Part model, mm, in its own coordinate system. A direction names the side the tool comes from. Give positions to 0.01 mm unless a question says otherwise; leave off trailing zeros. Answer in a Markdown table with one row per item. Add a question column.
1. Drop flat-ended pins along their axis: pin 1 Ø12 at (y, z) = (13, -27.5) entering from -X; pin 2 Ø2 at (x, y) = (-17, 9) entering from +Z; pin 3 Ø4 at (x, y) = (-11.5, 27.5) entering from +Z; pin 4 Ø1.5 at (x, z) = (-12.5, -30.5) entering from -Y. Give the stop position or say it passes through.
2. Probe line 1 along Z through (x, y) = (-9, 12); line 2 along X through (y, z) = (16, 34); line 3 along X through (y, z) = (32, 9). List the from-to ranges inside material, lowest first.
3. Band-saw the part on A-A on y = 12. State how many separate pieces and enclosed holes the cut face has, plus the area to 3 significant figures.
4. Which spindle directions (+Z, -Z, +X, -X, +Y, -Y) get a long thin tool onto all of the face, cutting with end or side? Do faces 1 (the flat face through (-3, 14, -25)), 2 (the flat face through (15, 15, -27)), 3 (the cylindrical face through (-24.08, 12.68, -13.28)), 4 (the flat face through (0, 25, 29)), 5 (the flat face through (0, 23, 30.35)). Say none if no direction does.
5. Pull direction Z, two halves, no side cores. Call faces 6 (the flat face through (3.61, 23.03, 32.45)), 7 (the flat face through (-15, 15, -27)), 8 (the conical face through (-1.036, 34.514, 24.386)): released by +Z, released by -Z, zero draft, split by the parting line, or undercut.
```python
from build123d import *

# Parameters (mm, degrees)
SKETCH2_W               = 6
SKETCH2_H               = 60
CUT_EXTRUDE1_DEPTH      = 67.520673478
CUT_EXTRUDE2_DEPTH      = 69.366658541
CUT_EXTRUDE2_DEPTH_BACK = 69.366658541
SKETCH3_R               = 4.25
SKETCH6_R               = 2.65
CUT_EXTRUDE5_DEPTH      = 67.520673599
CUT_EXTRUDE6_DEPTH      = 4
CUT_EXTRUDE7_DEPTH      = 62.846584554
FILLET1_R               = 28
SKETCH12_W              = 12
SKETCH12_H              = 3
BOSS_EXTRUDE1_DEPTH     = 25
CHAMFER1_SIZE           = 0.5
FILLET2_R               = 2
SKETCH13_R              = 4.625
CUT_EXTRUDE8_DEPTH      = 53.561734699
SKETCH15_R              = 2.65
BOSS_EXTRUDE2_DEPTH     = 0.2
SKETCH16_R              = 15
CUT_EXTRUDE9_DEPTH      = 55.660186193
FILLET3_R               = 11
FILLET4_R               = 24


with BuildPart() as part:
    # Sketch1 → Revolve1 (revolve)
    with BuildSketch(Plane.XY, mode=Mode.PRIVATE) as revolve1_sk:
        Polygon((16.25, 0), (40, 0), (40, 25), (27.5, 25), (24.25, 35), (16.25, 35), align=None)
    revolve(revolve1_sk.sketch.rotate(Axis((0, 0, 0), (0, 1, 0)), 90), axis=Axis((0, 0, 0), (0, 1, 0)))

    # Sketch2 → Cut-Extrude1 (cut, through all)
    with BuildSketch(Plane.XZ):
        with Locations((0, -30)):
            Rectangle(SKETCH2_W, SKETCH2_H)
    extrude(amount=-CUT_EXTRUDE1_DEPTH, mode=Mode.SUBTRACT)

    # Sketch3 → Cut-Extrude2 (cut, two sides: drawn at the far end of the back side and taken through both)
    with BuildSketch(Plane(origin=(-3, 0, 0), x_dir=(0, 0, -1), z_dir=(1, 0, 0)).offset(-CUT_EXTRUDE2_DEPTH_BACK)):
        with Locations((30.970676254, 12)):
            Circle(SKETCH3_R)
    extrude(amount=CUT_EXTRUDE2_DEPTH + CUT_EXTRUDE2_DEPTH_BACK, mode=Mode.SUBTRACT)

    # Sketch6 → Cut-Extrude5 (cut, through all)
    with BuildSketch(Plane.XZ):
        with Locations(Location((0, 34.5, 0), (0, 0, 270))):
            Circle(SKETCH6_R)
    extrude(amount=-CUT_EXTRUDE5_DEPTH, mode=Mode.SUBTRACT)

    # Sketch7 → Cut-Extrude6 (cut)
    with BuildSketch(Plane(origin=(0, 25, 0), x_dir=(1, 0, 0), z_dir=(0, 1, 0))):
        Polygon((-2.396003617, -30.35), (-4.792007234, -34.5), (-2.396003617, -38.65), (2.396003617, -38.65), (4.792007234, -34.5), (2.396003617, -30.35), align=None)
    extrude(amount=-CUT_EXTRUDE6_DEPTH, mode=Mode.SUBTRACT)

    # Sketch8 → Cut-Extrude7 (cut, through all)
    with BuildSketch(Plane(origin=(0, 25, 0), x_dir=(1, 0, 0), z_dir=(0, 1, 0))):
        with BuildLine():
            Line((-27.5, 0), (-27.5, -50))
            Line((-27.5, -50), (-50, -50))
            Line((-50, -50), (-50, 70))
            Line((-50, 70), (50, 70))
            Line((50, 70), (50, -50))
            Line((50, -50), (27.5, -50))
            Line((27.5, -50), (27.5, 0))
            ThreePointArc((27.5, 0), (24.173849507, 13.110110602), (15, 23.048861143))
            Line((15, 23.048861143), (15, 60))
            Line((15, 60), (-15, 60))
            Line((-15, 60), (-15, 23.048861143))
            ThreePointArc((-15, 23.048861143), (-24.173849507, 13.110110602), (-27.5, 0))
        make_face()
    extrude(amount=-CUT_EXTRUDE7_DEPTH, mode=Mode.SUBTRACT)

    # Fillet1
    # the kernel refuses this fillet: 28 mm, written as the material it takes off along each edge
    with BuildSketch(Plane(origin=(27.5, -77.857831737, 29.047375097), x_dir=(-0.9365360560407987, 0, 0.3505712705507198), z_dir=(0, 1, 0))) as fillet1_piece_1:
        with BuildLine():
            CenterArc((20.243036252, -25.791236836), FILLET1_R, 67.089723989, 92.388015463)
            Line((-5.979973318, -15.975241261), (0, 0))
            ThreePointArc((0, 0), (15.571566347, 3.155375949), (31.143132695, 0))
        make_face()
    extrude(amount=180.715663474, mode=Mode.SUBTRACT)
    with BuildSketch(Plane(origin=(-27.5, -77.857831737, 29.047375097), x_dir=(0, 0, -1), z_dir=(0, 1, 0))) as fillet1_piece_2:
        with BuildLine():
            CenterArc((17.057796288, -28), FILLET1_R, 90, 92.388015463)
            ThreePointArc((-10.917887598, -29.166666667), (-8.414067145, -13.477149178), (0, 0))
            Line((0, 0), (17.057796288, 0))
        make_face()
    extrude(amount=180.715663474, mode=Mode.SUBTRACT)

    # Sketch12 → Boss-Extrude1 (add)
    with BuildSketch(Plane(origin=(0, 25, 0), x_dir=(1, 0, 0), z_dir=(0, 1, 0))):
        with Locations((-9, 38.580992435)):
            Rectangle(SKETCH12_W, SKETCH12_H)
        with Locations((9, 38.580992435)):
            Rectangle(SKETCH12_W, SKETCH12_H)
    extrude(amount=-BOSS_EXTRUDE1_DEPTH)

    # Chamfer1
    chamfer1_edges = [part.edges().sort_by_distance(p)[0] for p in [
        (0, 0, 16.25),
    ]]
    chamfer(chamfer1_edges, length=CHAMFER1_SIZE)

    # Fillet2
    fillet2_edges = [part.edges().sort_by_distance(p)[0] for p in [
        (-15, 12.5, -40.080992435),
        (15, 12.5, -40.080992435),
    ]]
    fillet(fillet2_edges, radius=FILLET2_R)

    # Sketch13 → Cut-Extrude8 (cut, through all)
    with BuildSketch(Plane(origin=(0, 15, 0), x_dir=(1, 0, 0), z_dir=(0, 1, 0))):
        with Locations(Location((0, -34.5, 0), (0, 0, 270))):
            Circle(SKETCH13_R)
    extrude(amount=-CUT_EXTRUDE8_DEPTH, mode=Mode.SUBTRACT)

    # Sketch15 → Boss-Extrude2 (add)
    with BuildSketch(Plane.XZ.offset(-15)):
        with Locations(Location((0, 34.5, 0), (0, 0, 270))):
            Circle(SKETCH15_R)
    extrude(amount=-BOSS_EXTRUDE2_DEPTH)

    # Sketch16 → Cut-Extrude9 (cut, through all)
    with BuildSketch(Plane(origin=(0, 25, 0), x_dir=(1, 0, 0), z_dir=(0, 1, 0))):
        with Locations((25, -38)):
            Circle(SKETCH16_R)
        with Locations((-25, -38)):
            Circle(SKETCH16_R)
    extrude(amount=-CUT_EXTRUDE9_DEPTH, mode=Mode.SUBTRACT)

    # Fillet3
    fillet3_edges = [part.edges().sort_by_distance(p)[0] for p in [
        (10.000096358, 12.5, 37.946234534),
        (-10.000096358, 12.5, 37.946234534),
    ]]
    fillet(fillet3_edges, radius=FILLET3_R)

    # Fillet4
    fillet4_edges = [part.edges().sort_by_distance(p)[0] for p in [
        (-25.243486575, 12.5, 23.001976321),
        (25.243486575, 12.5, 23.001976321),
    ]]
    fillet(fillet4_edges, radius=FILLET4_R)


solid = part.part
```
Values:
| question | item | result |
|---|---|---|
| 1 | pin 1 | stops at x = -17.15 |
| 1 | pin 2 | stops at z = 26 |
| 1 | pin 3 | stops at z = 25.21 |
| 1 | pin 4 | stops at y = 0 |
| 2 | line 1 | z = -40.08 to -35.22, -26.72 to -13.53, 13.53 to 36.08 |
| 2 | line 2 | x = -10.4 to -2.6, 2.6 to 10.4 |
| 2 | line 3 | x = -23.56 to -13.53, 13.53 to 23.56 |
| 3 | separate pieces | 3 |
| 3 | enclosed holes | 1 |
| 3 | area | 1,950 mm² |
| 4 | face 1 | -Z, +Y, -Y |
| 4 | face 2 | -Z, +X, +Y, -Y |
| 4 | face 3 | -Z, -X, +Y, -Y |
| 4 | face 4 | +Z, +Y |
| 4 | face 5 | +Y |
| 5 | face 6 | undercut |
| 5 | face 7 | zero draft |
| 5 | face 8 | split by the parting line |
